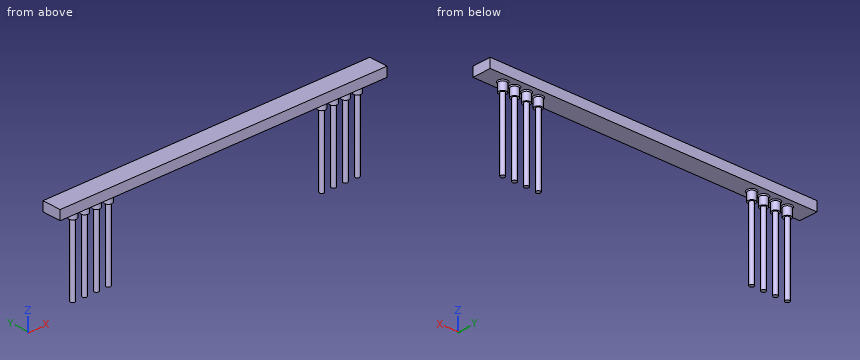
from build123d import *

# Parameters (mm, degrees)
SKETCH_W     = 70
SKETCH_H     = 4
PAD_DEPTH    = 2
SKETCH001_R  = 0.8
PAD001_DEPTH = 1.9
SKETCH002_R  = 0.475
PAD002_DEPTH = 15
CHAMFER_SIZE = 0.2


with BuildPart() as part:
    # Sketch → Pad (new body)
    with BuildSketch(Plane.XY):
        with Locations((0, -6.25)):
            Rectangle(SKETCH_W, SKETCH_H)
    extrude(amount=PAD_DEPTH)

    # Sketch001 (on Face5 of Pad) → Pad001 (join)
    with BuildSketch(Plane(origin=(0, 0, 0), x_dir=(1, 0, 0), z_dir=(0, 0, -1))):
        with Locations((-30.48, 6.25)):
            Circle(SKETCH001_R)
        with Locations((-22.86, 6.25)):
            Circle(SKETCH001_R)
        with Locations((-25.4, 6.25)):
            Circle(SKETCH001_R)
        with Locations((-27.94, 6.25)):
            Circle(SKETCH001_R)
        with Locations((22.86, 6.25)):
            Circle(SKETCH001_R)
        with Locations((25.4, 6.25)):
            Circle(SKETCH001_R)
        with Locations((27.94, 6.25)):
            Circle(SKETCH001_R)
        with Locations((30.48, 6.25)):
            Circle(SKETCH001_R)
    extrude(amount=PAD001_DEPTH)

    # Sketch002 (on Face17 of Pad001) → Pad002 (join)
    with BuildSketch(Plane(origin=(0, 0, -1.9), x_dir=(1, 0, 0), z_dir=(0, 0, -1))):
        with Locations((-30.48, 6.25)):
            Circle(SKETCH002_R)
        with Locations((-27.94, 6.25)):
            Circle(SKETCH002_R)
        with Locations((-25.4, 6.25)):
            Circle(SKETCH002_R)
        with Locations((-22.86, 6.25)):
            Circle(SKETCH002_R)
        with Locations((22.86, 6.25)):
            Circle(SKETCH002_R)
        with Locations((27.94, 6.25)):
            Circle(SKETCH002_R)
        with Locations((25.4, 6.25)):
            Circle(SKETCH002_R)
        with Locations((30.48, 6.25)):
            Circle(SKETCH002_R)
    extrude(amount=PAD002_DEPTH)

    # Chamfer
    chamfer_edges = [part.edges().sort_by_distance(p)[0] for p in [
        (-23.66, -6.25, 0),
        (-26.2, -6.25, 0),
        (-28.74, -6.25, 0),
        (-31.28, -6.25, 0),
        (22.06, -6.25, 0),
        (27.14, -6.25, 0),
        (24.6, -6.25, 0),
        (29.68, -6.25, 0),
    ]]
    chamfer(chamfer_edges, length=CHAMFER_SIZE)


solid = part.part
Read the model definition and answer for the solid it produces. Units are mm, in the model's axes. Round coordinates to 2 decimals unless told otherwise and drop trailing zeros. Loops run counter-clockwise (first coordinate to the right, second up) from the corner with the lowest first, then second, coordinate; pieces in that order, holes last.
Q1. This flat-tipped pin is pushed along its axis until it touches: pin 1 (2 mm diameter, centred on x = 15, y = -7.5, fed in from -Z). Where does it stop, or does it pass through?
Q2. Section A-A on z = -13.5 is taken. Write down the section's boundary in (x, y) (3 decimals).
Q3. Section B-B on z = -1 is taken. Write down the section's boundary in (x, y), and give its area (3 significant figures).
Q4. Consider probe 1 along Z at (x, y) = (17, -4.4); probe 2 along Y at (x, z) = (23, -12.25). Determine where each line is inside the solid, lowest interval first.
Q5. Section C-C on x = 1 is taken. Write down the section's boundary in (y, z), and give its area (3 significant figures).
Output:
1. pin 1: stops at z = 0
2. outline: circle Ø0.95 at (-30.48, -6.25); circle Ø0.95 at (-27.94, -6.25); circle Ø0.95 at (-25.4, -6.25); circle Ø0.95 at (-22.86, -6.25); circle Ø0.95 at (22.86, -6.25); circle Ø0.95 at (25.4, -6.25); circle Ø0.95 at (27.94, -6.25); circle Ø0.95 at (30.48, -6.25)
3. outline: circle Ø1.6 at (-30.48, -6.25); circle Ø1.6 at (-27.94, -6.25); circle Ø1.6 at (-25.4, -6.25); circle Ø1.6 at (-22.86, -6.25); circle Ø1.6 at (22.86, -6.25); circle Ø1.6 at (25.4, -6.25); circle Ø1.6 at (27.94, -6.25); circle Ø1.6 at (30.48, -6.25)
3. area: 16.1 mm2
4. probe 1: z = 0 to 2
4. probe 2: y = -6.7 to -5.8
5. outline: (-8.25, 0) - (-4.25, 0) - (-4.25, 2) - (-8.25, 2) - close
5. area: 8.00 mm2
